Verification items for the finished model (mm, model axes). A direction names the side the tool comes from. Round coordinates to 2 decimals unless told otherwise and drop trailing zeros. Order: outer loops, then holes, each group sorted by start corner. A loop starts at its lowest first (then second) coordinate and runs counter-clockwise, first axis right, second up. Notation, with made-up numbers: (54, 74.25) -> (88, 74.25) arc R28 ccw to (88, 111.25) -> close; hole circle Ø10 at (15.5, -7). An arc over 180 degrees is marked (long way). Answer in a Markdown table with one row per item. Add a question column.
```python
from build123d import *

# Parameters (mm, degrees)
BOSS_EXTRUDE1_DEPTH = 45
FILLET1_R           = 10
BOSS_EXTRUDE4_START = 3
BOSS_EXTRUDE4_DEPTH = 3
FILLET2_R           = 10


with BuildPart() as part:
    # Sketch1 → Boss-Extrude1 (new body)
    with BuildSketch(Plane(origin=(0, 0, 0), x_dir=(1, 0, 0), z_dir=(0, 1, 0))):
        with BuildLine():
            Line((-7, 16.039014932), (-7, 27.870533206))
            Line((-7, 27.870533206), (-2, 27.870533206))
            Line((-2, 27.870533206), (-2, 18.870533206))
            Line((-2, 18.870533206), (-2, 12.870533206))
            ThreePointArc((-2, 12.870533206), (0, -13.025), (2, 12.870533206))
            Line((2, 12.870533206), (2, 18.870533206))
            Line((2, 18.870533206), (2, 27.870533206))
            Line((2, 27.870533206), (7, 27.870533206))
            Line((7, 27.870533206), (7, 16.039014932))
            ThreePointArc((7, 16.039014932), (16.396088806, 6.117047643), (15.794877567, -7.534709195))
            ThreePointArc((15.794877567, -7.534709195), (16.882152496, -13.822605417), (22.097186029, -17.5))
            Line((22.097186029, -17.5), (35, -17.5))
            Line((35, -17.5), (35, -24.5))
            Line((35, -24.5), (27, -24.5))
            Line((27, -24.5), (27, -22.5))
            Line((27, -22.5), (31, -22.5))
            Line((31, -22.5), (31, -19.5))
            Line((31, -19.5), (-31, -19.5))
            Line((-31, -19.5), (-31, -22.5))
            Line((-31, -22.5), (-27, -22.5))
            Line((-27, -22.5), (-27, -24.5))
            Line((-27, -24.5), (-35, -24.5))
            Line((-35, -24.5), (-35, -17.5))
            Line((-35, -17.5), (-22.097186029, -17.5))
            ThreePointArc((-22.097186029, -17.5), (-16.882152496, -13.822605417), (-15.794877567, -7.534709195))
            ThreePointArc((-15.794877567, -7.534709195), (-16.396088806, 6.117047643), (-7, 16.039014932))
        make_face()
    extrude(amount=BOSS_EXTRUDE1_DEPTH)

    # Fillet1
    fillet1_edges = [part.edges().sort_by_distance(p)[0] for p in [
        (-2, 22.5, -12.870533206),
        (2, 22.5, -12.870533206),
    ]]
    fillet(fillet1_edges, radius=FILLET1_R)

    # Sketch3 → Boss-Extrude4 (add)
    with BuildSketch(Plane.XZ.offset(BOSS_EXTRUDE4_START)):
        with BuildLine():
            Line((-35, 24.5), (35, 24.5))
            Line((35, 24.5), (35, 17.5))
            Line((35, 17.5), (22.097186029, 17.5))
            ThreePointArc((22.097186029, 17.5), (16.882152496, 13.822605417), (15.794877567, 7.534709195))
            ThreePointArc((15.794877567, 7.534709195), (16.396088806, -6.117047643), (7, -16.039014932))
            Line((7, -16.039014932), (7, -27.870533206))
            Line((7, -27.870533206), (2, -27.870533206))
            Line((2, -27.870533206), (2, -19.650715636))
            ThreePointArc((2, -19.650715636), (3.27883999, -14.757723905), (6.788273616, -11.116202873))
            ThreePointArc((6.788273616, -11.116202873), (0, 13.025), (-6.788273616, -11.116202873))
            ThreePointArc((-6.788273616, -11.116202873), (-3.27883999, -14.757723905), (-2, -19.650715636))
            Line((-2, -19.650715636), (-2, -27.870533206))
            Line((-2, -27.870533206), (-7, -27.870533206))
            Line((-7, -27.870533206), (-7, -16.039014932))
            ThreePointArc((-7, -16.039014932), (-16.396088806, -6.117047643), (-15.794877567, 7.534709195))
            ThreePointArc((-15.794877567, 7.534709195), (-16.882152496, 13.822605417), (-22.097186029, 17.5))
            Line((-22.097186029, 17.5), (-35, 17.5))
            Line((-35, 17.5), (-35, 24.5))
        make_face()
    extrude(amount=-BOSS_EXTRUDE4_DEPTH)

    # Fillet2
    fillet2_edges = [part.edges().sort_by_distance(p)[0] for p in [
        (7, 22.5, -16.039014932),
        (-7, 22.5, -16.039014932),
    ]]
    fillet(fillet2_edges, radius=FILLET2_R)


solid = part.part
```
1) Cross-section at A-A, the plane z = 0.5. Record the boundary of the cut face in (x, y), and give its area (3 significant figures).
2) Cross-section at D-D, the plane y = 37. Record the boundary of the cut face in (x, z) (3 decimals).
3) Cross-section at C-C, the plane z = -20.5. Record the boundary of the cut face in (x, y).
4) Cross-section at B-B, the plane x = -14. Record the boundary of the cut face in (y, z).
5) Draft check along Z on faces 1 (the face through (-2, 21, -24)), 2 (the face through (-17.002, 20.664, -4.144)), 3 (the face through (-8.033, 21.336, -17.19)). Enter one of: +Z half, -Z half, draft (parallel to the pull), parting line (faces both ways), or undercut.
6) Thickness scan on L1, parallel to X at y = 25, z = 0 (3 decimals); L2, parallel to Z at x = 29, y = 4; L3, parallel to X at y = 5.5, z = 21. Record the ranges inside material, lowest first. Write a range as [from, to].
7) Tool access check on faces 4 (the face through (-7, 21, -25)), 5 (the face through (2, 21, -24)), 6 (the face through (-7.9, -0.4, 24.5)), 7 (the face through (29, 22, 22.5)), 8 (the face through (-27, 22, 23)). Record the directions out of +Z, -Z, +X, -X, +Y, -Y that give a thin tool (end or side, any length) a straight path to the whole face; none if there is none.
8) Depth check by flat-ended pin: P1, Ø4, axis at x = -9.5, z = 23, coming from the +Y side; P2, Ø8, axis at x = -10, y = 32.5, coming from the -Z side; P3, Ø4.5, axis at x = -28, y = 13.5, coming from the -Z side; P4, Ø4, axis at y = 11.5, z = -1, coming from the -X side. Enter the tip coordinate at first touch or a pass-through.
Results below:
| question | item | result |
|---|---|---|
| 1 | outline | (-17.49, -3) -> (-13.02, -3) -> (-13.02, 45) -> (-17.49, 45) -> close; (13.02, -3) -> (17.49, -3) -> (17.49, 45) -> (13.02, 45) -> close |
| 1 | area | 430 mm² |
| 2 | outline | (-35, 17.5) -> (-22.097, 17.5) arc R8.337 cw to (-15.795, 7.535) arc R17.5 ccw to (-10.818, -13.756) arc R10 cw to (-7, -21.616) -> (-7, -27.871) -> (-2, -27.871) -> (-2, -19.651) arc R10 ccw to (-6.788, -11.116) arc R13.025 cw (long way) to (6.788, -11.116) arc R10 ccw to (2, -19.651) -> (2, -27.871) -> (7, -27.871) -> (7, -21.616) arc R10 cw to (10.818, -13.756) arc R17.5 ccw to (15.795, 7.535) arc R8.337 cw to (22.097, 17.5) -> (35, 17.5) -> (35, 24.5) -> (27, 24.5) -> (27, 22.5) -> (31, 22.5) -> (31, 19.5) -> (-31, 19.5) -> (-31, 22.5) -> (-27, 22.5) -> (-27, 24.5) -> (-35, 24.5) -> close |
| 3 | outline | (-7.06, -3) -> (-2, -3) -> (-2, 45) -> (-7.06, 45) -> close; (2, -3) -> (7.06, -3) -> (7.06, 45) -> (2, 45) -> close |
| 4 | outline | (-3, -10.5) -> (45, -10.5) -> (45, 19.5) -> (0, 19.5) -> (0, 24.5) -> (-3, 24.5) -> close |
| 5 | face 1 | draft |
| 5 | face 2 | undercut |
| 5 | face 3 | -Z half |
| 6 | L1 | [-17.5, -13.025], [13.025, 17.5] |
| 6 | L2 | [17.5, 19.5], [22.5, 24.5] |
| 6 | L3 | [-35, -31], [31, 35] |
| 7 | face 4 | -Z, -X, +Y, -Y |
| 7 | face 5 | -Z, +Y, -Y |
| 7 | face 6 | +Z, +X, -X, +Y, -Y |
| 7 | face 7 | +Y |
| 7 | face 8 | +Z, +Y |
| 8 | P1 | y = 0 |
| 8 | P2 | z = -27.87 |
| 8 | P3 | z = 17.5 |
| 8 | P4 | x = -17.5 |
